from build123d import *

# Parameters (mm, degrees)
SKETCH_1_R          = 2
SKETCH_1_R_2        = 11.1
SKETCH_1_R_3        = 4.5
EXTRUDE_1_DEPTH     = 4
CUT_EXTRUDE_1_DEPTH = 95.135988932
FILLET_2_R          = 3


with BuildPart() as part:
    # 草图1 → 凸台-拉伸1 (new body)
    with BuildSketch(Plane(origin=(0, 0, 0), x_dir=(1, 0, 0), z_dir=(0, 1, 0))):
        with BuildLine():
            Line((-60, -24.852813742), (-21.213203436, -63.639610307))
            ThreePointArc((-21.213203436, -63.639610307), (0, -72.426406871), (21.213203436, -63.639610307))
            Line((21.213203436, -63.639610307), (60, -24.852813742))
            Line((60, -24.852813742), (60, 0))
            ThreePointArc((60, 0), (0, 60), (-60, 0))
            Line((-60, 0), (-60, -24.852813742))
        make_face()
        with Locations(Location((-28.25, 48.930435314, 0), (0, 0, 270))):
            Circle(SKETCH_1_R, mode=Mode.SUBTRACT)
        with Locations(Location((28.25, 48.930435314, 0), (0, 0, 270))):
            Circle(SKETCH_1_R, mode=Mode.SUBTRACT)
        with Locations(Location((56.5, 0, 0), (0, 0, 270))):
            Circle(SKETCH_1_R, mode=Mode.SUBTRACT)
        with Locations(Location((28.25, -48.930435314, 0), (0, 0, 270))):
            Circle(SKETCH_1_R, mode=Mode.SUBTRACT)
        with Locations(Location((0, 0, 0), (0, 0, 270))):
            Circle(SKETCH_1_R_2, mode=Mode.SUBTRACT)
        with Locations(Location((-28.25, -48.930435314, 0), (0, 0, 270))):
            Circle(SKETCH_1_R, mode=Mode.SUBTRACT)
        with Locations(Location((-56.5, 0, 0), (0, 0, 270))):
            Circle(SKETCH_1_R, mode=Mode.SUBTRACT)
        with Locations(Location((0, 29, 0), (0, 0, 270))):
            Circle(SKETCH_1_R, mode=Mode.SUBTRACT)
        with Locations(Location((25.11473671, -14.5, 0), (0, 0, 270))):
            Circle(SKETCH_1_R, mode=Mode.SUBTRACT)
        with Locations(Location((-25.11473671, -14.5, 0), (0, 0, 270))):
            Circle(SKETCH_1_R, mode=Mode.SUBTRACT)
        with Locations(Location((0, 19, 0), (0, 0, 270))):
            Circle(SKETCH_1_R_3, mode=Mode.SUBTRACT)
        with Locations(Location((-16.454482672, 9.5, 0), (0, 0, 270))):
            Circle(SKETCH_1_R_3, mode=Mode.SUBTRACT)
    extrude(amount=EXTRUDE_1_DEPTH)

    # 草图2 → 切除-拉伸1 (cut, through all)
    with BuildSketch(Plane(origin=(0, 4, 0), x_dir=(1, 0, 0), z_dir=(0, 1, 0))):
        with BuildLine():
            Line((-29.974316263, 44.917038689), (-17.928655829, 24.053342807))
            ThreePointArc((-17.928655829, 24.053342807), (-25.980762114, 15), (-29.795133831, 3.5))
            Line((-29.795133831, 3.5), (-53.886454699, 3.5))
            ThreePointArc((-53.886454699, 3.5), (-46.765371804, 27), (-29.974316263, 44.917038689))
        make_face()
        with BuildLine():
            Line((23.912138436, 48.417038689), (13.87859766, 31.038436285))
            ThreePointArc((13.87859766, 31.038436285), (0, 34), (-13.87859766, 31.038436285))
            Line((-13.87859766, 31.038436285), (-23.912138436, 48.417038689))
            ThreePointArc((-23.912138436, 48.417038689), (0, 54), (23.912138436, 48.417038689))
        make_face()
        with BuildLine():
            Line((53.886454699, 3.5), (29.795133831, 3.5))
            ThreePointArc((29.795133831, 3.5), (25.980762114, 15), (17.928655829, 24.053342807))
            Line((17.928655829, 24.053342807), (29.974316263, 44.917038689))
            ThreePointArc((29.974316263, 44.917038689), (46.765371804, 27), (53.886454699, 3.5))
        make_face()
        with BuildLine():
            Line((29.974316263, -44.917038689), (19.940775486, -27.538436285))
            ThreePointArc((19.940775486, -27.538436285), (29.444863729, -17), (33.819373146, -3.5))
            Line((33.819373146, -3.5), (53.886454699, -3.5))
            ThreePointArc((53.886454699, -3.5), (46.765371804, -27), (29.974316263, -44.917038689))
        make_face()
        with BuildLine():
            Line((-23.912138436, -48.417038689), (-11.866478002, -27.553342807))
            ThreePointArc((-11.866478002, -27.553342807), (0, -30), (11.866478002, -27.553342807))
            Line((11.866478002, -27.553342807), (23.912138436, -48.417038689))
            ThreePointArc((23.912138436, -48.417038689), (0, -54), (-23.912138436, -48.417038689))
        make_face()
        with BuildLine():
            Line((-53.886454699, -3.5), (-33.819373146, -3.5))
            ThreePointArc((-33.819373146, -3.5), (-29.444863729, -17), (-19.940775486, -27.538436285))
            Line((-19.940775486, -27.538436285), (-29.974316263, -44.917038689))
            ThreePointArc((-29.974316263, -44.917038689), (-46.765371804, -27), (-53.886454699, -3.5))
        make_face()
    extrude(amount=-CUT_EXTRUDE_1_DEPTH, mode=Mode.SUBTRACT)

    # 圆角2
    fillet_2_edges = [part.edges().sort_by_distance(p)[0] for p in [
        (29.974316263, 2, -44.917038689),
        (53.886454699, 2, -3.5),
        (29.795133831, 2, -3.5),
        (17.928655829, 2, -24.053342807),
        (19.940775486, 2, 27.538436285),
        (33.819373146, 2, 3.5),
        (53.886454699, 2, 3.5),
        (29.974316263, 2, 44.917038689),
        (13.87859766, 2, -31.038436285),
        (-13.87859766, 2, -31.038436285),
        (-23.912138436, 2, -48.417038689),
        (23.912138436, 2, -48.417038689),
        (-29.974316263, 2, 44.917038689),
        (-53.886454699, 2, 3.5),
        (-33.819373146, 2, 3.5),
        (-19.940775486, 2, 27.538436285),
        (-53.886454699, 2, -3.5),
        (-29.974316263, 2, -44.917038689),
        (-17.928655829, 2, -24.053342807),
        (-29.795133831, 2, -3.5),
        (23.912138436, 2, 48.417038689),
        (-23.912138436, 2, 48.417038689),
        (-11.866478002, 2, 27.553342807),
        (11.866478002, 2, 27.553342807),
    ]]
    fillet(fillet_2_edges, radius=FILLET_2_R)


solid = part.part
Work out the finished part from the listing and answer in its coordinate system (mm). Round coordinates to 2 decimals unless told otherwise and drop trailing zeros. Loops run counter-clockwise (first coordinate to the right, second up) from the corner with the lowest first, then second, coordinate; pieces in that order, holes last. Notation, with made-up numbers: (-38, 23.25) - (-20, 23.25) arc R14 cw to (-20, 41.25) - close; hole circle Ø1 at (62.25, 78). An arc over 180 degrees is marked (long way). One line per item, written item: value.
Q1. Find section C-C on x = 48. Give the vertices of the cut face in (y, z).
Check values:
outline: (0, -36) - (4, -36) - (4, -24.74) - (0, -24.74) - close; (0, -3.5) - (4, -3.5) - (4, 3.5) - (0, 3.5) - close; (0, 24.74) - (4, 24.74) - (4, 36.85) - (0, 36.85) - close
Q2. Each of these flat-tipped pins is pushed along its axis until it touches: pin 1 Ø3 at (x, z) = (0, -29) entering from +Y; pin 2 Ø1.2 at (x, y) = (-41, 2.5) entering from -Z; pin 3 Ø5 at (x, z) = (56.5, 0) entering from -Y; pin 4 Ø1.2 at (x, y) = (42.5, 1) entering from +Z. Where does it stop, or does it pass through?
Check values:
pin 1: through
pin 2: z = -44.36
pin 3: y = 0
pin 4: z = 42.95
Q3. Find section B-B on z = -29. Give the vertices of the cut face in (x, y).
Check values:
outline: (-52.53, 0) - (-45.55, 0) - (-45.55, 4) - (-52.53, 4) - close; (-20.78, 0) - (-2, 0) - (-2, 4) - (-20.78, 4) - close; (2, 0) - (20.78, 0) - (20.78, 4) - (2, 4) - close; (45.55, 0) - (52.53, 0) - (52.53, 4) - (45.55, 4) - close
Q4. Straight lines are drawn through the part: probe 1 along X at (y, z) = (2.95, 5); probe 2 along X at (y, z) = (1.9, 14.5); probe 3 along X at (y, z) = (2.8, 35.5). For each, find the intervals that lie inside material, in ascending order.
Check values:
probe 1: -60 to -53.18, -33.83 to -9.91, 9.91 to 33.83, 53.18 to 60
probe 2: -60 to -52.02, -30.75 to -27.11, -23.11 to 23.11, 27.11 to 30.75, 52.02 to 60
probe 3: -49.35 to -40.69, -24.54 to -16.45, 16.45 to 24.54, 40.69 to 49.35
Q5. Find section A-A on x = 0. Give the vertices of the cut face in (y, z).
Check values:
outline: (0, -60) - (4, -60) - (4, -54) - (0, -54) - close; (0, -34) - (4, -34) - (4, -31) - (0, -31) - close; (0, -27) - (4, -27) - (4, -23.5) - (0, -23.5) - close; (0, -14.5) - (4, -14.5) - (4, -11.1) - (0, -11.1) - close; (0, 11.1) - (4, 11.1) - (4, 30) - (0, 30) - close; (0, 54) - (4, 54) - (4, 72.43) - (0, 72.43) - close
Q6. The mould has two halves that part along Z. Classify faces 1 (the cylindrical face through (0, 2, -54)), 2 (the flat face through (-60, 2, 12)): +Z half, -Z half, draft (parallel to the pull), parting line (faces both ways), or undercut.
Check values:
face 1: undercut
face 2: draft
Q7. Find section D-D on z = -9.5. Give the vertices of the cut face in (x, y), and give its area (3 significant figures).
Check values:
outline: (-59.24, 0) - (-53.16, 0) - (-53.16, 4) - (-59.24, 4) - close; (-28.46, 0) - (-20.95, 0) - (-20.95, 4) - (-28.46, 4) - close; (-11.95, 0) - (-5.74, 0) - (-5.74, 4) - (-11.95, 4) - close; (5.74, 0) - (28.46, 0) - (28.46, 4) - (5.74, 4) - close; (53.16, 0) - (59.24, 0) - (59.24, 4) - (53.16, 4) - close
area: 194 mm2
